CAD build for the part. Positions are in the model's coordinates, mm. Give positions to 0.01 mm unless a question says otherwise; leave off trailing zeros. Order: outer loops, then holes, each group sorted by start corner. A loop starts at its lowest first (then second) coordinate and runs counter-clockwise, first axis right, second up. Notation, with made-up numbers: (-28.5, 24.5) -> (8.5, 24.5) arc R10 ccw to (8.5, 32.5) -> close; hole circle Ø2 at (36.5, 60). An arc over 180 degrees is marked (long way). Use one line per item in the form item = value. Start each with the question number.
1) Probe line 1 (X direction, y = 4, z = -282); line 2 (Z direction, x = 264, y = 3) (3 decimals); line 3 (Z direction, x = 241, y = 5.25) (3 decimals). List the from-to ranges inside material, lowest first.
2) Mould opens along Z. For faces 1 (the face through (67, 0, -270)), 2 (the face through (5.43, 3.22, -5.73)), 3 (the face through (209, 3.175, -445)) say: pulls with the +Z half, pulls with the -Z half, needs draft (parallel to the pull), parting line crosses it, or undercut.
3) Cut at B-B, the plane z = -434. Give the cut face in (x, y) (3 decimals).
4) Cut at C-C, the plane x = 223.5. Give the cut face in (y, z) (3 decimals).
from build123d import *

# Parameters (mm, degrees)
SKETCH1_W             = 419.1
SKETCH1_H             = 533.4
SKETCH1_W_2           = 246.0625
SKETCH1_H_2           = 346.075
OVERALL_SHAPE_DEPTH   = 6.35
SKETCH5_W             = 258.7625
SKETCH5_H             = 358.775
GLASS_INSET_CUT_DEPTH = 3.175
GLASS_INSET_FILLETS_R = 1.5875
FILLET1_R             = 19.05


with BuildPart() as part:
    # Sketch1 → Overall shape (new body)
    with BuildSketch(Plane(origin=(0, 0, 0), x_dir=(1, 0, 0), z_dir=(0, 1, 0))):
        with Locations((209.55, 266.7)):
            Rectangle(SKETCH1_W, SKETCH1_H)
        with Locations((209.55, 271.4625)):
            Rectangle(SKETCH1_W_2, SKETCH1_H_2, mode=Mode.SUBTRACT)
    extrude(amount=OVERALL_SHAPE_DEPTH)

    # Sketch5 → Glass inset cut (cut)
    with BuildSketch(Plane(origin=(0, 6.35, 0), x_dir=(1, 0, 0), z_dir=(0, 1, 0))):
        with Locations((209.55, 271.4625)):
            Rectangle(SKETCH5_W, SKETCH5_H)
    extrude(amount=-GLASS_INSET_CUT_DEPTH, mode=Mode.SUBTRACT)

    # Glass inset fillets
    glass_inset_fillets_edges = [part.edges().sort_by_distance(p)[0] for p in [
        (332.58125, 1.5875, -444.5),
        (86.51875, 1.5875, -444.5),
        (332.58125, 1.5875, -98.425),
        (86.51875, 1.5875, -98.425),
        (80.16875, 4.7625, -92.075),
        (80.16875, 4.7625, -450.85),
        (338.93125, 4.7625, -450.85),
        (338.93125, 4.7625, -92.075),
    ]]
    fillet(glass_inset_fillets_edges, radius=GLASS_INSET_FILLETS_R)

    # Fillet1
    fillet1_edges = [part.edges().sort_by_distance(p)[0] for p in [
        (419.1, 3.175, 0),
        (0, 3.175, 0),
    ]]
    fillet(fillet1_edges, radius=FILLET1_R)


solid = part.part
Result:
q1.line_1 = 0 to 80.17, 338.93 to 419.1
q1.line_2 = -533.4 to -444.5, -98.425 to 0
q1.line_3 = -533.4 to -450.85, -92.075 to 0
q2.face_1 = needs draft
q2.face_2 = pulls with the +Z half
q2.face_3 = undercut
q3.outline = (0, 0) -> (86.519, 0) -> (86.519, 3.175) -> (80.169, 3.175) -> (80.169, 6.35) -> (0, 6.35) -> close; (332.581, 0) -> (419.1, 0) -> (419.1, 6.35) -> (338.931, 6.35) -> (338.931, 3.175) -> (332.581, 3.175) -> close
q4.outline = (0, -533.4) -> (6.35, -533.4) -> (6.35, -450.85) -> (3.175, -450.85) -> (3.175, -444.5) -> (0, -444.5) -> close; (0, -98.425) -> (3.175, -98.425) -> (3.175, -92.075) -> (6.35, -92.075) -> (6.35, 0) -> (0, 0) -> close
